```python
from build123d import *

# Parameters (mm, degrees)
ESQUISSE17_R        = 1.5
BOSS_EXTRU_17_DEPTH = 3


with BuildPart() as part:
    # Esquisse17 → Boss.-Extru.17 (new body)
    with BuildSketch(Plane.XY):
        with BuildLine():
            Line((26.73219077, -35.312471899), (63.748376396, -35.312471899))
            ThreePointArc((63.748376396, -35.312471899), (65.869696739, -36.191151555), (66.748376396, -38.312471899))
            Line((66.748376396, -38.312471899), (66.748376396, -56.312471899))
            ThreePointArc((66.748376396, -56.312471899), (65.869696739, -58.433792242), (63.748376396, -59.312471899))
            Line((63.748376396, -59.312471899), (26.73219077, -59.312471899))
            ThreePointArc((26.73219077, -59.312471899), (24.610870426, -58.433792242), (23.73219077, -56.312471899))
            Line((23.73219077, -56.312471899), (23.73219077, -38.312471899))
            ThreePointArc((23.73219077, -38.312471899), (24.610870426, -36.191151555), (26.73219077, -35.312471899))
        make_face()
        with Locations((26.73219077, -38.312471899)):
            Circle(ESQUISSE17_R, mode=Mode.SUBTRACT)
        with Locations((63.748376396, -38.312471899)):
            Circle(ESQUISSE17_R, mode=Mode.SUBTRACT)
        with Locations((63.748376396, -56.312471899)):
            Circle(ESQUISSE17_R, mode=Mode.SUBTRACT)
        with Locations((26.73219077, -56.312471899)):
            Circle(ESQUISSE17_R, mode=Mode.SUBTRACT)
        with Locations((36.748376396, -38.312471899)):
            Circle(ESQUISSE17_R, mode=Mode.SUBTRACT)
        with Locations((36.748376396, -56.312471899)):
            Circle(ESQUISSE17_R, mode=Mode.SUBTRACT)
        Polygon((44.248376396, -41.312471899), (44.248376396, -38.312471899), (56.248376396, -38.312471899), (56.248376396, -41.312471899), (61.748376396, -41.312471899), (61.748376396, -53.312471899), (56.248376396, -53.312471899), (56.248376396, -56.312471899), (44.248376396, -56.312471899), (44.248376396, -53.312471899), (38.748376396, -53.312471899), (38.748376396, -41.312471899), align=None, mode=Mode.SUBTRACT)
    extrude(amount=BOSS_EXTRU_17_DEPTH)


solid = part.part
```
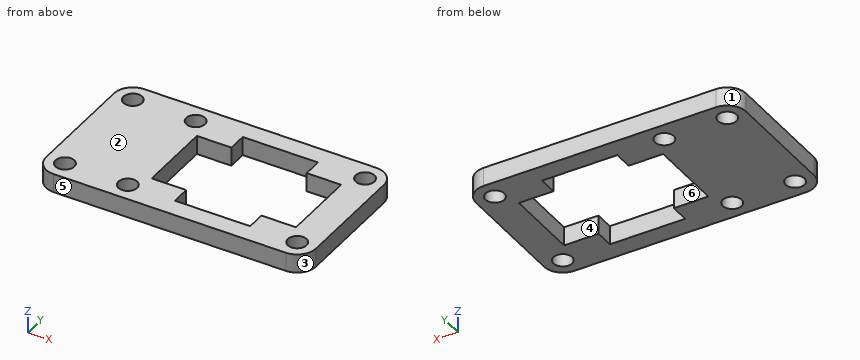
Here's how the part is built. I have some questions about the finished solid (model axes, mm). Face numbers are marked on the shaded views. A direction names the side the tool comes from. Give positions to 0.01 mm unless a question says otherwise; leave off trailing zeros. Order: outer loops, then holes, each group sorted by start corner. A loop starts at its lowest first (then second) coordinate and runs counter-clockwise, first axis right, second up. Notation, with made-up numbers: M -6,52.5 L 4,52.5 A16 cw 4,81.5 Z; hole C -10,85 d5. An arc over 180 degrees is marked long. Use a Markdown table: item, result. Add a question column.
1. Suppose I cut it at C-C (z = 2). List the corners of the cut face in (x, y) for me, and give its area (3 significant figures).
2. Suppose I cut it at D-D (y = -37.25). List the corners of the cut face in (x, z) for me, and give its area (3 significant figures).
3. Suppose I cut it at B-B (x = 59). List the corners of the cut face in (y, z) for me.
4. Suppose I cut it at A-A (y = -49.5). List the corners of the cut face in (x, z) for me, and give its area (3 significant figures).
5. If we mould it in two halves opening along Y, with no side actions, what happens to the marked faces 1, 2, 3 and 4? For each: +Y half, -Y half, draft (parallel to the pull), parting line (faces both ways), or undercut.
6. I need wall thicknesses on probe 1 along X at (y, z) = (-56.25, 1.65); probe 2 along Y at (x, z) = (56.5, 2.55); probe 3 along X at (y, z) = (-38.5, 1.75). Which ranges of each line are inside material? Lowest first, please. Write a range as from..to.
7. On a 3-axis mill with a long thin cutter (end or side, diameter ignored), from which of +Z, -Z, +X, -X, +Y, -Y can I reach the whole of each face in a straight line? I mean the marked faces 5 and 6. Say none if no direction works.
Results list:
| question | item | result |
|---|---|---|
| 1 | outline | M 23.73,-56.31 A3 ccw 26.73,-59.31 L 63.75,-59.31 A3 ccw 66.75,-56.31 L 66.75,-38.31 A3 ccw 63.75,-35.31 L 26.73,-35.31 A3 ccw 23.73,-38.31 Z; hole C 26.73,-56.31 d3; hole C 26.73,-38.31 d3; hole C 36.75,-56.31 d3; hole C 36.75,-38.31 d3; hole M 38.75,-53.31 L 44.25,-53.31 L 44.25,-56.31 L 56.25,-56.31 L 56.25,-53.31 L 61.75,-53.31 L 61.75,-41.31 L 56.25,-41.31 L 56.25,-38.31 L 44.25,-38.31 L 44.25,-41.31 L 38.75,-41.31 Z; hole C 63.75,-56.31 d3; hole C 63.75,-38.31 d3 |
| 1 | area | 634 mm² |
| 2 | outline | M 23.93,0 L 25.67,0 L 25.67,3 L 23.93,3 Z; M 27.79,0 L 35.69,0 L 35.69,3 L 27.79,3 Z; M 37.81,0 L 62.69,0 L 62.69,3 L 37.81,3 Z; M 64.81,0 L 66.55,0 L 66.55,3 L 64.81,3 Z |
| 2 | area | 109 mm² |
| 3 | outline | M -59.31,0 L -53.31,0 L -53.31,3 L -59.31,3 Z; M -41.31,0 L -35.31,0 L -35.31,3 L -41.31,3 Z |
| 4 | outline | M 23.73,0 L 38.75,0 L 38.75,3 L 23.73,3 Z; M 61.75,0 L 66.75,0 L 66.75,3 L 61.75,3 Z |
| 4 | area | 60.0 mm² |
| 5 | face 1 | +Y half |
| 5 | face 2 | draft |
| 5 | face 3 | -Y half |
| 5 | face 4 | undercut |
| 6 | probe 1 | x = 23.73..25.23, 28.23..35.25, 38.25..44.25, 56.25..62.25, 65.25..66.75 |
| 6 | probe 2 | y = -59.31..-53.31, -41.31..-35.31 |
| 6 | probe 3 | x = 23.73..25.24, 28.22..35.26, 38.24..44.25, 56.25..62.26, 65.24..66.75 |
| 7 | face 5 | +Z, -Z, +X, -X, -Y |
| 7 | face 6 | +Z, -Z |
